Can you work these out from the model? Positions are in its coordinate system, mm. A direction names the side the tool comes from. Round coordinates to 2 decimals unless told otherwise and drop trailing zeros. Order: outer loops, then holes, each group sorted by start corner. A loop starts at its lowest first (then second) coordinate and runs counter-clockwise, first axis right, second up. Notation, with made-up numbers: (34, 10.25) -> (54, 10.25) arc R11 ccw to (54, 16.25) -> close; hole circle Ø5 at (51, 52.5). An arc over 180 degrees is marked (long way). One line per item, written item: value.
Autodesk Inventor part; units mm, degrees
ref_plane "YZ Plane" through (0, 0, 0) normal (1, 0, 0) x (0, 1, 0)
ref_plane "XZ Plane" through (0, 0, 0) normal (0, 1, 0) x (-1, 0, 0)
ref_plane "XY Plane" through (0, 0, 0) normal (0, 0, 1) x (1, 0, 0)
sketch "Sketch1" plane through (0, 0, 0) normal (0, 1, 0) x (-1, 0, 0)
  circle A0 centre (0, 0) radius 57.5
  dimension "d0" = 115
extrude "Extrusion1" add sketch "Sketch1" along normal blind 660
sketch "Sketch2" plane through (0, 660, 0) normal (0, 1, 0) x (1, 0, 0)
  circle A0 centre (0, 0) radius 20
  dimension "d3" = 40
extrude "Extrusion2" add sketch "Sketch2" along normal blind 40
fillet "Fillet1" radius 50 1 edges at (57.5, 660, 0)
properties part number "Cylinder"
Q1. Will these pins go through, and if not, where does the flat tip stop? pin 1 Ø1.5 at (x, z) = (-25.5, -16) entering from -Y; pin 2 Ø4 at (y, z) = (629.5, 27) entering from +X; pin 3 Ø1 at (y, z) = (469, -35) entering from +X; pin 4 Ø6 at (x, z) = (-23.5, 31) entering from +Y.
Answers below:
pin 1: y = 0
pin 2: x = 48.36
pin 3: x = 46
pin 4: y = 652.74
Q2. I want a section at A-A on y = 161.5. List the corners of the cut face in (x, z) for me, plus the area to 3 significant figures.
Answers below:
outline: circle Ø115 at (0, 0)
area: 10,400 mm^2
Q3. Please list where these lines run through material, in increasing order: line 1 along X through (y, z) = (228, 0.5); line 2 along Z through (x, y) = (3, 419.5); line 3 along X through (y, z) = (139, 3.5).
Answers below:
line 1: -57.5 to 57.5
line 2: -57.42 to 57.42
line 3: -57.39 to 57.39
Q4. On a 3-axis mill with a long thin cutter (end or side, diameter ignored), from which of +Z, -Z, +X, -X, +Y, -Y can I reach the whole of each face in a straight line? I mean faces 1 (the face through (-4.336, 679.72, -19.524)), 2 (the face through (12.465, 301.513, 56.133)). Say none if no direction works.
Answers below:
face 1: +Y
face 2: +Y, -Y
